Verification items for the finished model (mm, model axes). A direction names the side the tool comes from. Coordinates: 2 decimals unless noted, no trailing zeros. Write each loop counter-clockwise with the first axis right and the second up, starting at its lowest first coordinate (ties: lowest second). Pieces come first, ordered by that corner, then holes. Notation, with made-up numbers: (18.5, 32.25) -> (71.5, 32.25) arc R12 ccw to (71.5, 52.25) -> close; hole circle Ø6 at (59, 0). An arc over 180 degrees is marked (long way). Use a Markdown table: item, result. Add a question column.
from build123d import *

# Parameters (mm, degrees)
IZIM1_R                     = 20.65
Y_KSEKLIK_EKSTR_ZYON1_DEPTH = 6
KES_EKSTR_ZYON1_START       = -6
KES_EKSTR_ZYON1_DEPTH       = 6
IZIM4_R                     = 8.66
KES_EKSTR_ZYON2_DEPTH       = 6


with BuildPart() as part:
    # Çizim1 → Yükseklik-Ekstrüzyon1 (new body)
    with BuildSketch(Plane.XY):
        Circle(IZIM1_R)
    extrude(amount=Y_KSEKLIK_EKSTR_ZYON1_DEPTH)

    # Çizim3 → Kes-Ekstrüzyon1 (cut)
    with BuildSketch(Plane.XY.offset(6).offset(KES_EKSTR_ZYON1_START)):
        with BuildLine():
            Line((8.04, 14.865005886), (8.04, 19.020538899))
            ThreePointArc((8.04, 19.020538899), (20.65, 0), (8.04, -19.020538899))
            Line((8.04, -19.020538899), (8.04, -14.865005886))
            ThreePointArc((8.04, -14.865005886), (16.9, 0), (8.04, 14.865005886))
        make_face()
        with BuildLine():
            Line((-8.04, 14.865005886), (-8.04, 19.020538899))
            ThreePointArc((-8.04, 19.020538899), (-20.65, 0), (-8.04, -19.020538899))
            Line((-8.04, -19.020538899), (-8.04, -14.865005886))
            ThreePointArc((-8.04, -14.865005886), (-16.9, 0), (-8.04, 14.865005886))
        make_face()
    extrude(amount=KES_EKSTR_ZYON1_DEPTH, mode=Mode.SUBTRACT)

    # Çizim4 → Kes-Ekstrüzyon2 (cut)
    with BuildSketch(Plane.XY.offset(6)):
        Circle(IZIM4_R)
    extrude(amount=-KES_EKSTR_ZYON2_DEPTH, mode=Mode.SUBTRACT)


solid = part.part
1) Cross-section at A-A on y = 0. Record the boundary of the cut face in (x, z).
2) Gauge pin test, flat ends, axial feed: pin 1 (14 mm diameter, centred on x = 0, y = 0, fed in from +Z); pin 2 (2 mm diameter, centred on y = 9, z = 0.5, fed in from -X); pin 3 (1.2 mm diameter, centred on y = 17.5, z = 1.5, fed in from -X); pin 4 (3.5 mm diameter, centred on y = -17.5, z = 4.5, fed in from +X). Record the tip position at first contact, or that the pin passes through.
3) Cross-section at C-C on z = 4.5. Record the boundary of the cut face in (x, y) (3 decimals).
4) Cross-section at D-D on x = -11. Record the boundary of the cut face in (y, z).
5) Cross-section at B-B on x = 0. Record the boundary of the cut face in (y, z), then the cut area to 3 significant figures.
6) Thickness scan on L1, parallel to Y at x = 0, z = 2.85; L2, parallel to Y at x = 4.5, z = 0.35; L3, parallel to X at y = 19, z = 2.7. Record the ranges inside material, lowest first.
7) Release check for a two-part mould opening along Y. For faces 1 (the face through (16.9, -0.25, 2.96)), 2 (the face through (-8, 5, 0)), 3 (the face through (-6.87, -5.27, 3.04)) record: released by +Y, released by -Y, zero draft, split by the parting line, or undercut.
8) Set-up check for faces 4 (the face through (-8.04, 17, 3)), 5 (the face through (-8, 5, 6)), 6 (the face through (8.04, 17, 3)), 7 (the face through (-8.04, -17, 3)), 8 (the face through (8.04, -17, 3)): record each of +Z, -Z, +X, -X, +Y, -Y from which the full face is reachable in a straight line by a thin tool's end or side.
Returned:
| question | item | result |
|---|---|---|
| 1 | outline | (-16.9, 0) -> (-8.66, 0) -> (-8.66, 6) -> (-16.9, 6) -> close; (8.66, 0) -> (16.9, 0) -> (16.9, 6) -> (8.66, 6) -> close |
| 2 | pin 1 | passes through |
| 2 | pin 2 | stops at x = -14.89 |
| 2 | pin 3 | stops at x = -8.04 |
| 2 | pin 4 | stops at x = 8.04 |
| 3 | outline | (-8.04, -19.021) arc R20.65 ccw to (8.04, -19.021) -> (8.04, -14.865) arc R16.9 ccw to (8.04, 14.865) -> (8.04, 19.021) arc R20.65 ccw to (-8.04, 19.021) -> (-8.04, 14.865) arc R16.9 ccw to (-8.04, -14.865) -> close; hole circle Ø17.32 at (0, 0) |
| 4 | outline | (-12.83, 0) -> (12.83, 0) -> (12.83, 6) -> (-12.83, 6) -> close |
| 5 | outline | (-20.65, 0) -> (-8.66, 0) -> (-8.66, 6) -> (-20.65, 6) -> close; (8.66, 0) -> (20.65, 0) -> (20.65, 6) -> (8.66, 6) -> close |
| 5 | area | 144 mm² |
| 6 | L1 | y = -20.65 to -8.66, 8.66 to 20.65 |
| 6 | L2 | y = -20.15 to -7.4, 7.4 to 20.15 |
| 6 | L3 | x = -8.04 to 8.04 |
| 7 | face 1 | split by the parting line |
| 7 | face 2 | zero draft |
| 7 | face 3 | undercut |
| 8 | face 4 | +Z, -Z, -X, +Y |
| 8 | face 5 | +Z, +X, -X, +Y, -Y |
| 8 | face 6 | +Z, -Z, +X, +Y |
| 8 | face 7 | +Z, -Z, -X, -Y |
| 8 | face 8 | +Z, -Z, +X, -Y |
